Source: CAD feature listing. Evaluate the final solid. Frame: model axes, mm. Face numbers are marked on the shaded views. A direction names the side the tool comes from. Give positions to 0.01 mm unless a question says otherwise; leave off trailing zeros. Order: outer loops, then holes, each group sorted by start corner. A loop starts at its lowest first (then second) coordinate and runs counter-clockwise, first axis right, second up.
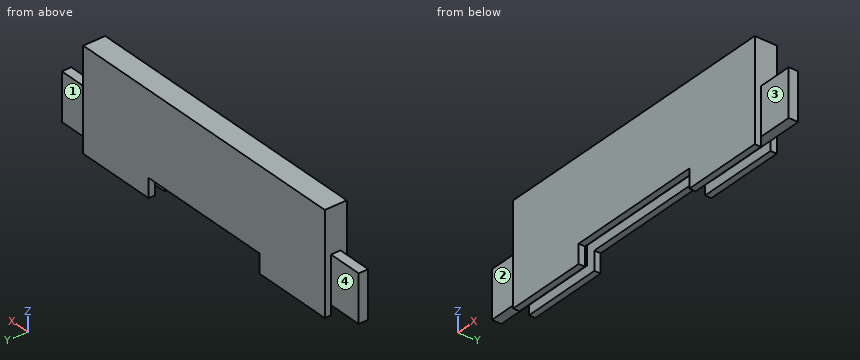
from build123d import *

# Parameters (mm, degrees)
F1_DEPTH = 22.225
F2_W     = 34.925
F2_H     = 6.35
F3_DEPTH = 57.15
F2_H_2   = 9.525
F2_W_2   = 73.025
F2_W_3   = 158.75
F4_DEPTH = 9.525
F5_DEPTH = 28.575


with BuildPart() as f1:
    # F0 (on Front) → F1 (new body)
    with BuildSketch(Plane.XZ):
        Polygon((0, 57.15), (0, 0), (117.475, 0), (117.475, 19.05), (257.175, 19.05), (257.175, 0), (374.65, 0), (374.65, 57.15), (339.725, 57.15), (339.725, 101.6), (34.925, 101.6), (34.925, 57.15), align=None)
    extrude(amount=F1_DEPTH)

    # F2 (on Top) → F3 (cut, through all)
    with BuildSketch(Plane.XY):
        with Locations((357.1875, -19.05)):
            Rectangle(F2_W, F2_H)
        with Locations((357.1875, -3.175)):
            Rectangle(F2_W, F2_H)
        with Locations((17.4625, -19.05)):
            Rectangle(F2_W, F2_H)
        with Locations((17.4625, -3.175)):
            Rectangle(F2_W, F2_H)
    extrude(amount=F3_DEPTH, mode=Mode.SUBTRACT)

    # F2 (on Top) → F4 (cut)
    with BuildSketch(Plane.XY):
        with Locations((17.4625, -11.1125)):
            Rectangle(F2_W, F2_H_2)
        with Locations((71.4375, -11.1125)):
            Rectangle(F2_W_2, F2_H_2)
        with Locations((357.1875, -11.1125)):
            Rectangle(F2_W, F2_H_2)
        with Locations((303.2125, -11.1125)):
            Rectangle(F2_W_2, F2_H_2)
        with Locations((187.325, -11.1125)):
            Rectangle(F2_W_3, F2_H_2)
    extrude(amount=F4_DEPTH, mode=Mode.SUBTRACT)

    # F2 (on Top) → F5 (cut)
    with BuildSketch(Plane.XY):
        with Locations((187.325, -11.1125)):
            Rectangle(F2_W_3, F2_H_2)
    extrude(amount=F5_DEPTH, mode=Mode.SUBTRACT)


solid = f1.part
1) First-contact query: pin 1 Ø5 at (x, y) = (345, -9) entering from -Z (3 decimals); pin 2 Ø7 at (x, y) = (162, -2) entering from -Z; pin 3 Ø1.9 at (y, z) = (-19, 9) entering from +X (3 decimals). Flat tips, straight axial feed; report the tip coordinate or a pass-through.
Checks:
pin 1: stops at z = 9.525
pin 2: stops at z = 19.05
pin 3: stops at x = 339.725
2) Section query C-C on x = 336. Output: boundary loops of the cut face in (y, z) (3 decimals), and give its area (3 significant figures).
Checks:
outline: (-22.225, 0) - (-15.875, 0) - (-15.875, 9.525) - (-6.35, 9.525) - (-6.35, 0) - (0, 0) - (0, 101.6) - (-22.225, 101.6) - close
area: 2,170 mm2
3) Reachability of the marked faces 1, 2, 3 and 4 from +Z, -Z, +X, -X, +Y, -Y: full face, straight path, thin tool, end or side. Return the list, or none.
Checks:
face 1: +Z, -Z, +X, +Y
face 2: +Z, -Z, -X, -Y
face 3: +Z, -Z, +X, -Y
face 4: +Z, -Z, -X, +Y
4) Ray query, L1, parallel to X at y = -8.5, z = 27; L2, parallel to X at y = -5.5, z = 59 (3 decimals); L3, parallel to Y at x = 182, z = 20 (3 decimals). Return the intervals inside material, ascending.
Checks:
L1: x = 0 to 107.95, 266.7 to 374.65
L2: x = 34.925 to 339.725
L3: y = -22.225 to -15.875, -6.35 to 0
5) Section query D-D on x = 161.5. Output: boundary loops of the cut face in (y, z) (3 decimals), and give its area (3 significant figures).
Checks:
outline: (-22.225, 19.05) - (-15.875, 19.05) - (-15.875, 28.575) - (-6.35, 28.575) - (-6.35, 19.05) - (0, 19.05) - (0, 101.6) - (-22.225, 101.6) - close
area: 1,740 mm2
6) Section query B-B on z = 45. Output: boundary loops of the cut face in (x, y) (3 decimals).
Checks:
outline: (0, -15.875) - (34.925, -15.875) - (34.925, -22.225) - (339.725, -22.225) - (339.725, -15.875) - (374.65, -15.875) - (374.65, -6.35) - (339.725, -6.35) - (339.725, 0) - (34.925, 0) - (34.925, -6.35) - (0, -6.35) - close
7) Section query A-A on y = -12. Output: boundary loops of the cut face in (x, z) (3 decimals).
Checks:
outline: (0, 9.525) - (107.95, 9.525) - (107.95, 28.575) - (266.7, 28.575) - (266.7, 9.525) - (374.65, 9.525) - (374.65, 57.15) - (339.725, 57.15) - (339.725, 101.6) - (34.925, 101.6) - (34.925, 57.15) - (0, 57.15) - close
